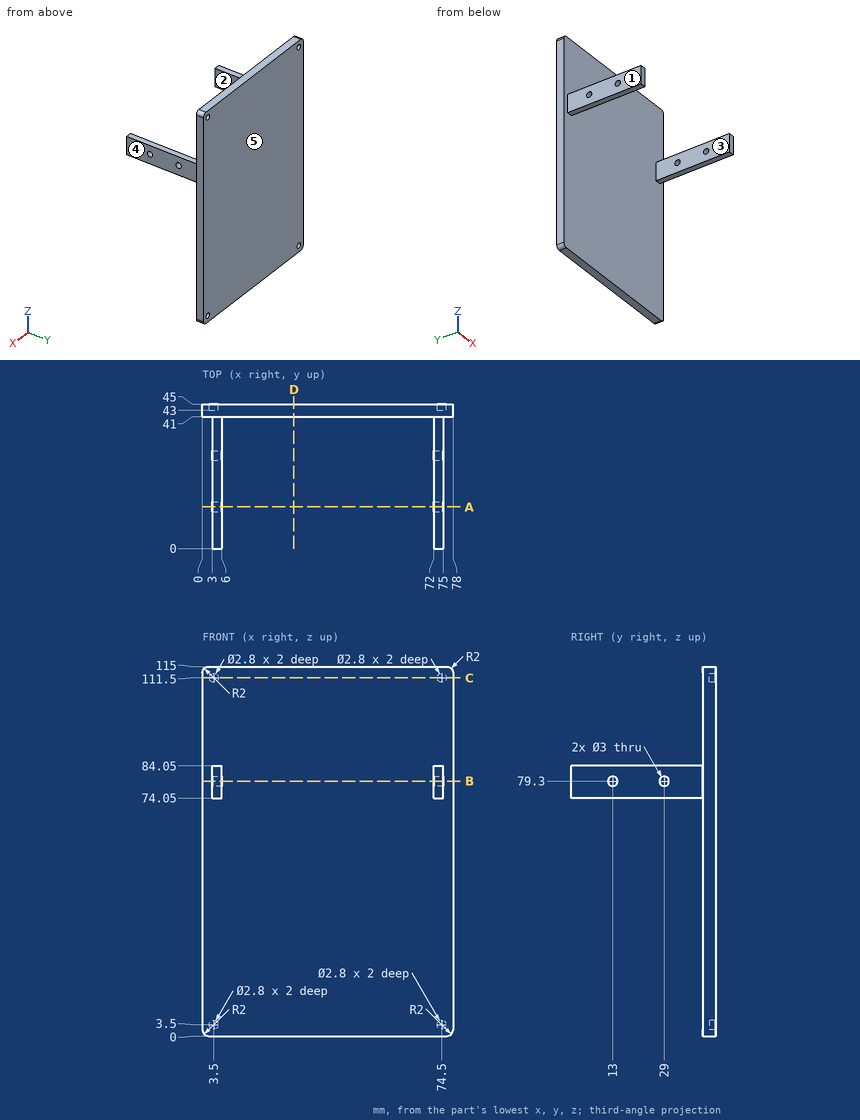
Geometry check sheet. Reference: drawing and pictorial views, mm from the part's lowest x, y, z. A direction names the side the tool comes from. Coordinates: 2 decimals unless noted, no trailing zeros. Write each loop counter-clockwise with the first axis right and the second up, starting at its lowest first coordinate (ties: lowest second). Pieces come first, ordered by that corner, then holes. Notation, with made-up numbers: M 53.5,-9 L 95.5,-9 A6 cw 95.5,1 Z; hole C -30.5,81.5 d5. An arc over 180 degrees is marked long. One line per question, with ' | ' between items.
1) Sectioned sample at D-D on x = 28.5. Record the cut outline in (y, z).
Solutions:
outline: M 41,0 L 45,0 L 45,115 L 41,115 Z
2) Material ranges on L1, parallel to Z at x = 74.5, y = 44.3; L2, parallel to Y at x = 4.3, z = 79.3; L3, parallel to Z at x = 74, y = 15, recorded low to high.
Solutions:
L1: 0 to 2.1, 4.9 to 110.1, 112.9 to 115 | L2: 0 to 11.5, 14.5 to 27.5, 30.5 to 45 | L3: 74.05 to 84.05
3) Sectioned sample at A-A on y = 13. Record the cut outline in (x, z), then the cut area to 3 significant figures.
Solutions:
outline: M 3,74.05 L 6,74.05 L 6,77.8 L 3,77.8 Z; M 3,80.8 L 6,80.8 L 6,84.05 L 3,84.05 Z; M 72,74.05 L 75,74.05 L 75,77.8 L 72,77.8 Z; M 72,80.8 L 75,80.8 L 75,84.05 L 72,84.05 Z | area: 42.0 mm^2
4) Access from +Z, -Z, +X, -X, +Y, -Y to the whole of each face (thin tool, end or side, straight path). Record for the marked faces 1 and 2.
Solutions:
face 1: +Z, -Z, -X, -Y | face 2: +Z, -Z, -Y
5) Sectioned sample at B-B on z = 79.3. Record the cut outline in (x, y).
Solutions:
outline: M 0,41 L 3,41 L 3,30.5 L 6,30.5 L 6,41 L 72,41 L 72,30.5 L 75,30.5 L 75,41 L 78,41 L 78,45 L 0,45 Z; M 3,0 L 6,0 L 6,11.5 L 3,11.5 Z; M 3,14.5 L 6,14.5 L 6,27.5 L 3,27.5 Z; M 72,0 L 75,0 L 75,11.5 L 72,11.5 Z; M 72,14.5 L 75,14.5 L 75,27.5 L 72,27.5 Z
6) Release check for a two-part mould opening along X. For the marked faces 3, 4 and 5 record: +X half, -X half, draft (parallel to the pull), parting line (faces both ways), or undercut.
Solutions:
face 3: undercut | face 4: +X half | face 5: draft
7) Sectioned sample at C-C on z = 111.5. Record the cut outline in (x, y), then the cut area to 3 significant figures.
Solutions:
outline: M 0,41 L 78,41 L 78,45 L 75.9,45 L 75.9,43 L 73.1,43 L 73.1,45 L 4.9,45 L 4.9,43 L 2.1,43 L 2.1,45 L 0,45 Z | area: 301 mm^2
8) Depth check by flat-ended pin: pin 1 Ø11 at (y, z) = (22.5, 76.5) entering from -X; pin 2 Ø0.8 at (x, z) = (74.5, 3) entering from +Y; pin 3 Ø0.9 at (x, y) = (4.5, 24) entering from -Z. Enter the tip coordinate at first touch or a pass-through.
Solutions:
pin 1: x = 3 | pin 2: y = 43 | pin 3: z = 74.05
